from build123d import *

# Parameters (mm, degrees)
EXTRUDE_2_DEPTH      = 19
EXTRUDE_3_DEPTH      = 40
CUT_EXTRUDE_START    = -32
CUT_EXTRUDE_1_DEPTH  = 32
SKETCH_4_R           = 4.1
CUT_EXTRUDE_2_DEPTH  = 60.916608716
EXTRUDE_4_REACH      = 102.922
EXTRUDE_4_END_RADIUS = 35
EXTRUDE_START        = -37
SKETCH_5_R           = 10
SKETCH_5_R_2         = 1.5
SKETCH_5_4_R         = 1.5
CUT_EXTRUDE_3_DEPTH  = 66.038450252
CUT_EXTRUDE_4_DEPTH  = 12
SKETCH_6_R           = 4
CUT_EXTRUDE_5_DEPTH  = 30
SKETCH_10_W          = 80
SKETCH_10_H          = 68
CUT_EXTRUDE_6_DEPTH  = 76.617458351
SKETCH_11_W          = 80
SKETCH_11_H          = 20
CUT_EXTRUDE_7_DEPTH  = 69.629439801
SKETCH_12_W          = 10
SKETCH_12_H          = 20
CUT_EXTRUDE_8_DEPTH  = 59.660037571
SKETCH_13_W          = 10
SKETCH_13_H          = 20
CUT_EXTRUDE_9_DEPTH  = 59.660037571
SKETCH_14_R          = 1.5
CUT_EXTRUDE_10_DEPTH = 64.000000016


with BuildPart() as part:
    # Эскиз1 → Бобышка-Вытянуть2 (new, symmetric)
    with BuildSketch(Plane.XY):
        with BuildLine():
            Line((35, 0), (26, 0))
            ThreePointArc((26, 0), (0, -26), (-26, 0))
            Line((-26, 0), (-35, 0))
            ThreePointArc((-35, 0), (0, -35), (35, 0))
        make_face()
        with BuildLine():
            Line((26, 0), (24, 0))
            ThreePointArc((24, 0), (0, -24), (-24, 0))
            Line((-24, 0), (-26, 0))
            ThreePointArc((-26, 0), (0, -26), (26, 0))
        make_face()
    extrude(amount=EXTRUDE_2_DEPTH, both=True)

    # Эскиз2 → Бобышка-Вытянуть3 (add)
    with BuildSketch(Plane(origin=(0, 0, 0), x_dir=(1, 0, 0), z_dir=(0, 1, 0))):
        with BuildLine():
            ThreePointArc((50, 0), (47.071067812, 7.071067812), (40, 10))
            ThreePointArc((40, 10), (37.411809549, 9.659258263), (35, 8.660254038))
            Line((35, 8.660254038), (35, -8.660254038))
            ThreePointArc((35, -8.660254038), (37.411809549, -9.659258263), (40, -10))
            ThreePointArc((40, -10), (47.071067812, -7.071067812), (50, 0))
        make_face()
        with BuildLine():
            Line((35, -8.660254038), (35, 8.660254038))
            ThreePointArc((35, 8.660254038), (31.339745962, 5), (30, 0))
            ThreePointArc((30, 0), (31.339745962, -5), (35, -8.660254038))
        make_face()
        with BuildLine():
            ThreePointArc((35, 8.660254038), (37.411809549, 9.659258263), (40, 10))
            Line((40, 10), (35, 10))
            Line((35, 10), (35, 8.660254038))
        make_face()
        with BuildLine():
            Line((35, -10), (40, -10))
            ThreePointArc((40, -10), (37.411809549, -9.659258263), (35, -8.660254038))
            Line((35, -8.660254038), (35, -10))
        make_face()
        with BuildLine():
            Line((35, 8.660254038), (35, 10))
            Line((35, 10), (30, 10))
            Line((30, 10), (30, 0))
            ThreePointArc((30, 0), (31.339745962, 5), (35, 8.660254038))
        make_face()
        with BuildLine():
            ThreePointArc((35, -8.660254038), (31.339745962, -5), (30, 0))
            Line((30, 0), (30, -10))
            Line((30, -10), (35, -10))
            Line((35, -10), (35, -8.660254038))
        make_face()
    extrude_3 = extrude(amount=-EXTRUDE_3_DEPTH)

    # Эскиз3 → Вырез-Вытянуть1 (cut)
    with BuildSketch(Plane.XZ.offset(40).offset(CUT_EXTRUDE_START)):
        with BuildLine():
            Line((40, 10), (30, 10))
            Line((30, 10), (30, -10))
            Line((30, -10), (40, -10))
            ThreePointArc((40, -10), (50, 0), (40, 10))
        make_face()
    cut_extrude_1 = extrude(amount=CUT_EXTRUDE_1_DEPTH, mode=Mode.SUBTRACT)

    # Эскиз4 → Вырез-Вытянуть2 (cut, through all)
    with BuildSketch(Plane.XZ.offset(8)):
        with Locations(Location((40, 0, 0), (0, 0, 270))):
            Circle(SKETCH_4_R)
    cut_extrude_2 = extrude(amount=-CUT_EXTRUDE_2_DEPTH, mode=Mode.SUBTRACT)

    # Зеркальное отражение1: Бобышка-Вытянуть3, Вырез-Вытянуть1, Вырез-Вытянуть2 across plane
    add(extrude_3.mirror(Plane(origin=(0, 0, 0), x_dir=(0, 0, 1), z_dir=(1, 0, 0))))
    add(cut_extrude_1.mirror(Plane(origin=(0, 0, 0), x_dir=(0, 0, 1), z_dir=(1, 0, 0))), mode=Mode.SUBTRACT)
    add(cut_extrude_2.mirror(Plane(origin=(0, 0, 0), x_dir=(0, 0, 1), z_dir=(1, 0, 0))), mode=Mode.SUBTRACT)

    # Бобышка-Вытянуть4: up to this cylinder (the profile starts outside it)
    extrude_4_end = Plane(origin=(0, 0, 4.8585785), z_dir=(0, 0, -1)) * Cylinder(EXTRUDE_4_END_RADIUS, 286.561157, mode=Mode.PRIVATE)
    # Эскиз5 → Бобышка-Вытянуть4 (add, up to the surface)
    with BuildSketch(Plane(origin=(0, 0, 0), x_dir=(1, 0, 0), z_dir=(0, 1, 0)).offset(EXTRUDE_START), mode=Mode.PRIVATE) as extrude_4_sk1:
        with Locations(Location((0, 0, 0), (0, 0, 90))):
            Circle(SKETCH_5_R)
        Circle(SKETCH_5_R_2, mode=Mode.SUBTRACT)
    extrude_4_tool1 = extrude(extrude_4_sk1.sketch, amount=EXTRUDE_4_REACH, mode=Mode.PRIVATE) - extrude_4_end
    add(extrude_4_tool1.solids().sort_by_distance((0, -37, 9.717157))[0])
    # Эскиз5 → Бобышка-Вытянуть4 (add, up to the surface)
    with BuildSketch(Plane(origin=(0, 0, 0), x_dir=(1, 0, 0), z_dir=(0, 1, 0)).offset(EXTRUDE_START), mode=Mode.PRIVATE) as extrude_4_sk2:
        Circle(SKETCH_5_R_2)
    extrude_4_tool2 = extrude(extrude_4_sk2.sketch, amount=EXTRUDE_4_REACH, mode=Mode.PRIVATE) - extrude_4_end
    add(extrude_4_tool2.solids().sort_by_distance((0, -37, 0))[0])

    # Эскиз5<4> → Вырез-Вытянуть3 (cut, through all)
    with BuildSketch(Plane(origin=(0, 0, 0), x_dir=(1, 0, 0), z_dir=(0, 1, 0))):
        with Locations(Location((0, 0, 0), (0, 0, 270))):
            Circle(SKETCH_5_4_R)
    extrude(amount=-CUT_EXTRUDE_3_DEPTH, mode=Mode.SUBTRACT)

    # Эскиз1<4> → Вырез-Вытянуть4 (cut, symmetric)
    with BuildSketch(Plane.XY):
        with BuildLine():
            ThreePointArc((-24, 0), (0, 24), (24, 0))
            Line((24, 0), (26, 0))
            ThreePointArc((26, 0), (0, 26), (-26, 0))
            Line((-26, 0), (-24, 0))
        make_face()
        with BuildLine():
            Line((26, 0), (24, 0))
            ThreePointArc((24, 0), (0, -24), (-24, 0))
            Line((-24, 0), (-26, 0))
            ThreePointArc((-26, 0), (0, -26), (26, 0))
        make_face()
    extrude(amount=CUT_EXTRUDE_4_DEPTH, both=True, mode=Mode.SUBTRACT)

    # Эскиз6 → Вырез-Вытянуть5 (cut)
    with BuildSketch(Plane(origin=(0, 0, 0), x_dir=(1, 0, 0), z_dir=(0, 1, 0))):
        with Locations(Location((0, 0, 0), (0, 0, 270))):
            Circle(SKETCH_6_R)
    extrude(amount=-CUT_EXTRUDE_5_DEPTH, mode=Mode.SUBTRACT)

    # Эскиз7 → Повернуть1 (revolve)
    with BuildSketch(Plane.XY):
        with BuildLine():
            Line((0, 33), (0, -33))
            ThreePointArc((0, -33), (33, 0), (0, 33))
        make_face()
    revolve(axis=Axis((0, 0, 0), (0, 1, 0)))

    # Эскиз8 → Вырез-Повернуть1 (revolve, cut)
    with BuildSketch(Plane.XY):
        with BuildLine():
            Line((0, 29), (0, -29))
            ThreePointArc((0, -29), (29, 0), (0, 29))
        make_face()
    revolve(axis=Axis((0, 0, 0), (0, 1, 0)), mode=Mode.SUBTRACT)

    # Эскиз10 → Вырез-Вытянуть6 (cut, through all)
    with BuildSketch(Plane(origin=(0, 0, -10), x_dir=(-1, 0, 0), z_dir=(0, 0, -1))):
        with Locations((0, -1)):
            Rectangle(SKETCH_10_W, SKETCH_10_H)
    cut_extrude_6 = extrude(amount=CUT_EXTRUDE_6_DEPTH, mode=Mode.SUBTRACT)

    # Зеркальное отражение2: Вырез-Вытянуть6 across plane
    add(cut_extrude_6.mirror(Plane.XY), mode=Mode.SUBTRACT)

    # Эскиз11 → Вырез-Вытянуть7 (cut, through all)
    with BuildSketch(Plane(origin=(0, 0, 0), x_dir=(1, 0, 0), z_dir=(0, 1, 0))):
        Rectangle(SKETCH_11_W, SKETCH_11_H)
    extrude(amount=CUT_EXTRUDE_7_DEPTH, mode=Mode.SUBTRACT)

    # Эскиз12 → Вырез-Вытянуть8 (cut, through all)
    with BuildSketch(Plane.XZ.offset(8)):
        with Locations((-35, 0)):
            Rectangle(SKETCH_12_W, SKETCH_12_H)
    extrude(amount=CUT_EXTRUDE_8_DEPTH, mode=Mode.SUBTRACT)

    # Эскиз13 → Вырез-Вытянуть9 (cut, through all)
    with BuildSketch(Plane.XZ.offset(8)):
        with Locations((35, 0)):
            Rectangle(SKETCH_13_W, SKETCH_13_H)
    extrude(amount=CUT_EXTRUDE_9_DEPTH, mode=Mode.SUBTRACT)

    # Эскиз14 → Вырез-Вытянуть10 (cut, through all)
    with BuildSketch(Plane.XZ.offset(37)):
        with Locations(Location((0, 0, 0), (0, 0, 90))):
            Circle(SKETCH_14_R)
    extrude(amount=-CUT_EXTRUDE_10_DEPTH, mode=Mode.SUBTRACT)


solid = part.part
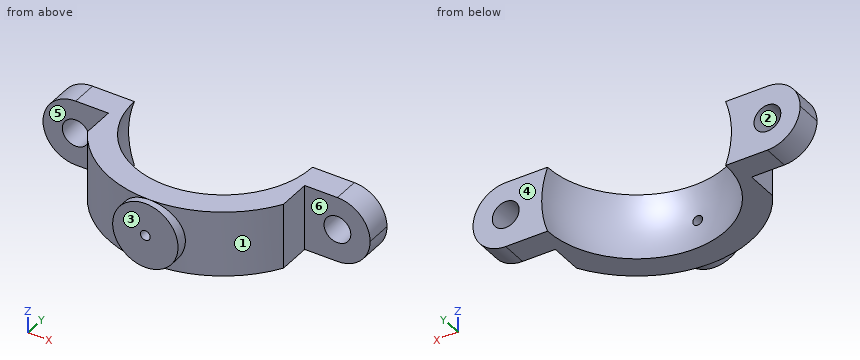
Check sheet for the modelled part. Datum: model origin and axes. Units: mm. Face numbers are marked on the shaded views. A direction names the side the tool comes from. Round coordinates to 2 decimals unless told otherwise and drop trailing zeros. Order: outer loops, then holes, each group sorted by start corner. A loop starts at its lowest first (then second) coordinate and runs counter-clockwise, first axis right, second up.
Q1. Cross-section at A-A, the plane x = 41.5. Enter the section's corners in (y, z), plus the area to 3 significant figures.
Filled sheet:
outline: (-8, -9.89) - (0, -9.89) - (0, -3.82) - (-8, -3.82) - close; (-8, 3.82) - (0, 3.82) - (0, 9.89) - (-8, 9.89) - close
area: 97.1 mm2
Q2. Cross-section at C-C, the plane x = 9. Enter the section's corners in (y, z).
Filled sheet:
outline: (-37, -4.36) - (-33.82, -4.36) - (-33.82, -10) - (-25.69, -10) arc R27.57 cw to (-25.69, 10) - (-33.82, 10) - (-33.82, 4.36) - (-37, 4.36) - close
Q3. Depth check by flat-ended pin: P1, Ø5, axis at y = -12, z = -1.5, coming from the -X side; P2, Ø2, axis at x = 29, z = -4.5, coming from the -Y side; P3, Ø8, axis at y = -12.5, z = -2.5, coming from the +X side. Enter the tip coordinate at first touch or a pass-through.
Filled sheet:
P1: stops at x = -30
P2: stops at y = -21
P3: stops at x = 30
Q4. Scan lines: L1, parallel to Z at x = 40, y = -2.75; L2, parallel to X at y = -33.75, z = 0; L3, parallel to Y at x = -34.5, z = 8. Record each from-to range of solid material in increasing order.
Filled sheet:
L1: z = -10 to -4.1, 4.1 to 10
L2: x = -10 to -1.5, 1.5 to 10
L3: y = -8 to 0
Q5. Draft check along X on the marked faces 1, 2 and 3. Enter one of: pulls with the +X half, pulls with the -X half, needs draft (parallel to the pull), parting line crosses it, or undercut.
Filled sheet:
face 1: pulls with the +X half
face 2: undercut
face 3: needs draft
Q6. Cross-section at B-B, the plane z = -6.75. Enter the section's corners in (x, y).
Filled sheet:
outline: (-47.38, -8) - (-30, -8) - (-30, -18.03) arc R35 ccw to (-7.38, -34.21) - (-7.38, -37) - (7.38, -37) - (7.38, -34.21) arc R35 ccw to (30, -18.03) - (30, -8) - (47.38, -8) - (47.38, 0) - (28.2, 0) arc R28.2 cw to (-28.2, 0) - (-47.38, 0) - close
Q7. Cross-section at D-D, the plane x = 21. Enter the section's corners in (y, z).
Filled sheet:
outline: (-28, -10) - (-17.32, -10) arc R20 cw to (-17.32, 10) - (-28, 10) - close
Q8. Set-up check for the marked faces 4, 5 and 6: record each of +Z, -Z, +X, -X, +Y, -Y from which the full face is reachable in a straight line by a thin tool's end or side.
Filled sheet:
face 4: +Z, -Z, +X, -X, +Y
face 5: +Z, -Z, -X, -Y
face 6: +Z, -Z, +X, -Y
